from build123d import *

# Parameters (mm, degrees)
CUT_EXTRUDE2_DEPTH      = 20.92888597
CUT_EXTRUDE2_DEPTH_BACK = 20.92888597
SKETCH2_3_R             = 1.7526
SKETCH2_3_R_2           = 1.4605
SKETCH2_R               = 1.7526
CUT_EXTRUDE1_DEPTH      = 3.556
FILLET1_R               = 0.635


with BuildPart() as part:
    # Sketch1 → Revolve1 (revolve)
    with BuildSketch(Plane.XY):
        Polygon((-14.986, 6.35), (-8.636, 6.35), (-8.636, 12.7), (-2.286, 12.7), (-2.286, 6.35), (0, 6.35), (0, 4), (-14.986, 4), align=None)
    revolve(axis=Axis((0, 0, 0), (-1, 0, 0)))

    # Sketch2_3 → Cut-Extrude2 (cut, two sides: drawn at the far end of the back side and taken through both)
    with BuildSketch(Plane.ZY.offset(8.636).offset(-CUT_EXTRUDE2_DEPTH_BACK)):
        with Locations(Location((-9.779, 0, 0), (0, 0, 270))):
            Circle(SKETCH2_3_R)
        with Locations(Location((0, 9.779, 0), (0, 0, 270))):
            Circle(SKETCH2_3_R)
        with Locations(Location((9.779, 0, 0), (0, 0, 270))):
            Circle(SKETCH2_3_R)
        with Locations(Location((0, -9.779, 0), (0, 0, 270))):
            Circle(SKETCH2_3_R)
        with Locations(Location((-6.914797213, 6.914797213, 0), (0, 0, 270))):
            Circle(SKETCH2_3_R_2)
        with Locations(Location((6.914797213, 6.914797213, 0), (0, 0, 270))):
            Circle(SKETCH2_3_R_2)
        with Locations(Location((6.914797213, -6.914797213, 0), (0, 0, 270))):
            Circle(SKETCH2_3_R_2)
        with Locations(Location((-6.914797213, -6.914797213, 0), (0, 0, 270))):
            Circle(SKETCH2_3_R_2)
    extrude(amount=CUT_EXTRUDE2_DEPTH + CUT_EXTRUDE2_DEPTH_BACK, mode=Mode.SUBTRACT)

    # Sketch2 → Cut-Extrude1 (cut)
    # profile 1 of 4: a face of its own
    with BuildSketch(Plane.ZY.offset(8.636)):
        with BuildLine():
            Line((-12.201800216, -3.52222536), (-9.249720354, -3.001694031))
            ThreePointArc((-9.249720354, -3.001694031), (-6.731, 0), (-9.249720354, 3.001694031))
            Line((-9.249720354, 3.001694031), (-12.201800216, 3.52222536))
            ThreePointArc((-12.201800216, 3.52222536), (-12.7, 0), (-12.201800216, -3.52222536))
        make_face()
        with Locations(Location((-9.779, 0, 0), (0, 0, 270))):
            Circle(SKETCH2_R, mode=Mode.SUBTRACT)
    # profile 2 of 4: a face of its own
    with BuildSketch(Plane.ZY.offset(8.636)):
        with BuildLine():
            Line((-3.001694031, -9.249720354), (-3.52222536, -12.201800216))
            ThreePointArc((-3.52222536, -12.201800216), (0, -12.7), (3.52222536, -12.201800216))
            Line((3.52222536, -12.201800216), (3.001694031, -9.249720354))
            ThreePointArc((3.001694031, -9.249720354), (0, -6.731), (-3.001694031, -9.249720354))
        make_face()
        with Locations(Location((0, -9.779, 0), (0, 0, 270))):
            Circle(SKETCH2_R, mode=Mode.SUBTRACT)
    # profile 3 of 4: a face of its own
    with BuildSketch(Plane.ZY.offset(8.636)):
        with BuildLine():
            ThreePointArc((3.52222536, 12.201800216), (0, 12.7), (-3.52222536, 12.201800216))
            Line((-3.52222536, 12.201800216), (-3.001694031, 9.249720354))
            ThreePointArc((-3.001694031, 9.249720354), (0, 6.731), (3.001694031, 9.249720354))
            Line((3.001694031, 9.249720354), (3.52222536, 12.201800216))
        make_face()
        with Locations(Location((0, 9.779, 0), (0, 0, 270))):
            Circle(SKETCH2_R, mode=Mode.SUBTRACT)
    # profile 4 of 4: a face of its own
    with BuildSketch(Plane.ZY.offset(8.636)):
        with BuildLine():
            Line((9.249720354, -3.001694031), (12.201800216, -3.52222536))
            ThreePointArc((12.201800216, -3.52222536), (12.7, 0), (12.201800216, 3.52222536))
            Line((12.201800216, 3.52222536), (9.249720354, 3.001694031))
            ThreePointArc((9.249720354, 3.001694031), (6.731, 0), (9.249720354, -3.001694031))
        make_face()
        with Locations(Location((9.779, 0, 0), (0, 0, 270))):
            Circle(SKETCH2_R, mode=Mode.SUBTRACT)
    extrude(amount=-CUT_EXTRUDE1_DEPTH, mode=Mode.SUBTRACT)

    # Fillet1
    fillet1_edges = [part.edges().sort_by_distance(p)[0] for p in [
        (-6.858, 12.201800216, -3.52222536),
        (-6.858, 12.201800216, 3.52222536),
        (-6.858, -3.52222536, -12.201800216),
        (-6.858, 3.52222536, -12.201800216),
        (-6.858, -12.201800216, 3.52222536),
        (-6.858, -12.201800216, -3.52222536),
        (-6.858, 3.52222536, 12.201800216),
        (-6.858, -3.52222536, 12.201800216),
    ]]
    fillet(fillet1_edges, radius=FILLET1_R)


solid = part.part
Input: part model. Units: mm. Frame: model coordinates. A direction names the side the tool comes from. Round coordinates to 2 decimals unless told otherwise and drop trailing zeros. Write each loop counter-clockwise with the first axis right and the second up, starting at its lowest first coordinate (ties: lowest second). Pieces come first, ordered by that corner, then holes.
1) Contact query for flat-ended pins moving along their axis: P1, Ø2.5, axis at y = 6.91, z = -6.91, coming from the +X side; P2, Ø8, axis at x = -11.5, y = 1, coming from the -Z side; P3, Ø1.8, axis at y = -1, z = -8.5, coming from the -X side; P4, Ø4, axis at x = -2.5, z = -9.5, coming from the +Y side. Output: stop coordinate, or through.
2) Cut plane D-D (x = -4). Count the separate pieces of the cut face and the enclosed holes in it, then the cut area to 3 significant figures.
3) Ray query, L1, parallel to Z at x = -3.25, y = 0; L2, parallel to Z at x = -9.25, y = -0.25. Return the intervals inside material, ascending.
4) Cut plane A-A (z = 0). Return the cut outline in (x, y).
5) Cut plane C-C (x = -11.25). Return the cut outline in (y, z), then the cut area to 3 significant figures.
6) Reachability of faces 5 (the flat face through (-6.88, -10.38, 3.2)), 6 (the cylindrical face through (-11.77, -1.38, 6.2)), 7 (the flat face through (-6.883, 3.196, -10.352)), 8 (the flat face through (-6.883, -3.196, 10.352)) from +Z, -Z, +X, -X, +Y, -Y: full face, straight path, thin tool, end or side. Return the list, or none.
7) Draft query along Y for faces 1 (the flat face through (-5.08, -12, 0)), 2 (the flat face through (-5.08, 0, -12)), 3 (the cylindrical face through (-3.663, 0.228, 11.517)), 4 (the cylindrical face through (-6.83, -11.93, 3.71)). Return one class per face: pulls with the +Y half, pulls with the -Y half, needs draft (parallel to the pull), parting line crosses it, or undercut.
Geometry says:
1. P1: passes through
1. P2: stops at z = -11.97
1. P3: stops at x = -5.08
1. P4: stops at y = 10.25
2. separate pieces: 1
2. enclosed holes: 9
2. area: 391 mm2
3. L1: z = -12.7 to -11.53, -8.03 to -4, 4 to 8.03, 11.53 to 12.7
3. L2: z = -6.35 to -3.99, 3.99 to 6.35
4. outline: (-14.99, -6.35) - (-8.64, -6.35) - (-8.64, -6.73) - (-5.08, -6.73) - (-5.08, -8.03) - (-2.29, -8.03) - (-2.29, -6.35) - (0, -6.35) - (0, -4) - (-14.99, -4) - close; (-14.99, 4) - (0, 4) - (0, 6.35) - (-2.29, 6.35) - (-2.29, 8.03) - (-5.08, 8.03) - (-5.08, 6.73) - (-8.64, 6.73) - (-8.64, 6.35) - (-14.99, 6.35) - close; (-5.08, -12.7) - (-2.29, -12.7) - (-2.29, -11.53) - (-5.08, -11.53) - close; (-5.08, 11.53) - (-2.29, 11.53) - (-2.29, 12.7) - (-5.08, 12.7) - close
5. outline: circle Ø12.7 at (0, 0); hole circle Ø8 at (0, 0)
5. area: 76.4 mm2
6. face 5: -X, -Y
6. face 6: -X
6. face 7: -Z, -X
6. face 8: +Z, -X
7. face 1: needs draft
7. face 2: undercut
7. face 3: undercut
7. face 4: pulls with the -Y half
